from build123d import *

# Parameters (mm, degrees)
BOSS_EXTRUDE1_DEPTH     = 9.525
FILLET1_R               = 25.4
BOSS_EXTRUDE2_DEPTH     = 19.05
FILLET2_R               = 6.35
CUT_EXTRUDE1_DEPTH      = 7.9375
SKETCH9_R               = 14.2875
CUT_EXTRUDE3_DEPTH      = 10.525
CUT_EXTRUDE3_DEPTH_BACK = 10.525


with BuildPart() as part:
    # Sketch1 → Boss-Extrude1 (new body, symmetric)
    with BuildSketch(Plane(origin=(0, 0, 0), x_dir=(0, 0, -1), z_dir=(1, 0, 0))):
        Polygon((0, 0), (0, -112.563749307), (261.582885953, -457.593888215), (450.85, -457.593888215), (450.85, 690.679166755), (208.861297127, 733.352902663), (171.366736958, 520.733599781), (293.482501466, 499.198975136), (217.390599948, 67.706860465), (221.513774593, 49.108421529), align=None)
    extrude(amount=BOSS_EXTRUDE1_DEPTH, both=True)

    # Fillet1
    fillet1_edges = [part.edges().sort_by_distance(p)[0] for p in [
        (0, 499.198975136, -293.482501466),
        (0, 520.733599781, -171.366736958),
        (0, 733.352902663, -208.861297127),
        (0, 690.679166755, -450.85),
        (0, -457.593888215, -450.85),
        (0, -457.593888215, -261.582885953),
        (0, -112.563749307, 0),
    ]]
    fillet(fillet1_edges, radius=FILLET1_R)

    # Sketch5 → Boss-Extrude2 (add)
    with BuildSketch(Plane(origin=(9.525, 0, 0), x_dir=(0, 0, -1), z_dir=(1, 0, 0))):
        Polygon((24.797918581, 5.497566194), (23.079929145, 13.246915751), (147.069522049, 40.734746721), (148.787511485, 32.985397164), align=None)
    extrude(amount=-BOSS_EXTRUDE2_DEPTH)

    # Fillet2
    fillet2_edges = [part.edges().sort_by_distance(p)[0] for p in [
        (0, 32.985397164, -148.787511485),
        (0, 5.497566194, -24.797918581),
    ]]
    fillet(fillet2_edges, radius=FILLET2_R)

    # Sketch6 → Cut-Extrude1 (cut)
    with BuildSketch(Plane(origin=(9.525, 0, 0), x_dir=(0, 0, -1), z_dir=(1, 0, 0))):
        with BuildLine():
            Line((28.6385, -6.365075015), (28.6385, -100.980075015))
            ThreePointArc((28.6385, -100.980075015), (20.574, -109.044575015), (12.5095, -100.980075015))
            Line((12.5095, -100.980075015), (12.5095, -6.365075015))
            ThreePointArc((12.5095, -6.365075015), (20.574, 1.699424985), (28.6385, -6.365075015))
        make_face()
        with BuildLine():
            Line((418.973, -269.390231885), (418.973, 670.409768115))
            ThreePointArc((418.973, 670.409768115), (427.0375, 678.474268115), (435.102, 670.409768115))
            Line((435.102, 670.409768115), (435.102, -269.390231885))
            ThreePointArc((435.102, -269.390231885), (427.0375, -277.454731885), (418.973, -269.390231885))
        make_face()
        with BuildLine():
            Line((354.524032203, 662.256458615), (332.470713639, 537.185873983))
            ThreePointArc((332.470713639, 537.185873983), (323.128345786, 530.644277587), (316.586749391, 539.98664544))
            Line((316.586749391, 539.98664544), (338.640067954, 665.057230073))
            ThreePointArc((338.640067954, 665.057230073), (347.982435807, 671.598826468), (354.524032203, 662.256458615))
        make_face()
        with BuildLine():
            Line((406.559861559, 491.68872453), (197.491872287, 528.553051841))
            ThreePointArc((197.491872287, 528.553051841), (189.629312583, 536.333399232), (194.145410605, 546.430849865))
            Line((194.145410605, 546.430849865), (228.335527156, 740.311741223))
            ThreePointArc((228.335527156, 740.311741223), (231.057354489, 742.217510482), (232.963123748, 739.495683149))
            Line((232.963123748, 739.495683149), (199.190848291, 547.984231028))
            Line((199.190848291, 547.984231028), (409.934019299, 510.824523979))
            ThreePointArc((409.934019299, 510.824523979), (417.814840153, 499.569545384), (406.559861559, 491.68872453))
        make_face()
        with BuildLine():
            Line((250.866088981, 80.873965121), (323.642040242, 493.606894408))
            ThreePointArc((323.642040242, 493.606894408), (317.100443846, 502.949262261), (307.758075993, 496.407665866))
            Line((307.758075993, 496.407665866), (234.982124733, 83.674736578))
            ThreePointArc((234.982124733, 83.674736578), (241.523721128, 74.332368726), (250.866088981, 80.873965121))
        make_face()
        with BuildLine():
            Line((41.2115, -97.692152626), (91.0115, -97.692152626))
            ThreePointArc((91.0115, -97.692152626), (99.076, -105.756652626), (91.0115, -113.821152626))
            Line((91.0115, -113.821152626), (41.2115, -113.821152626))
            ThreePointArc((41.2115, -113.821152626), (33.147, -105.756652626), (41.2115, -97.692152626))
        make_face()
    extrude(amount=-CUT_EXTRUDE1_DEPTH, mode=Mode.SUBTRACT)

    # Sketch9 → Cut-Extrude3 (cut, two sides)
    with BuildSketch(Plane(origin=(0, 0, 0), x_dir=(0, 0, -1), z_dir=(1, 0, 0))) as cut_extrude3_sk:
        with Locations((49.5935, -44.45)):
            Circle(SKETCH9_R)
    extrude(amount=CUT_EXTRUDE3_DEPTH, mode=Mode.SUBTRACT)
    extrude(cut_extrude3_sk.sketch, amount=-CUT_EXTRUDE3_DEPTH_BACK, mode=Mode.SUBTRACT)


solid = part.part
The model under review builds one solid part; all positions refer to its coordinate system, in mm. A direction names the side the tool comes from. Coordinates: 2 decimals unless noted, no trailing zeros. Write each loop counter-clockwise with the first axis right and the second up, starting at its lowest first coordinate (ties: lowest second). Pieces come first, ordered by that corner, then holes. Notation, with made-up numbers: M 35.5,-37.75 L 51.5,-37.75 A19 cw 51.5,-27.75 Z; hole C 46,-31 d10. An arc over 180 degrees is marked long. Put each result on its own line as item: value.
1) Draft analysis for pull direction Z (two halves, no side actions). For faces 4 (the flat face through (-9.525, 144, -272)), 5 (the flat face through (1.588, 290, -279)), 6 (the cylindrical face through (0.13, 685.88, -444.75)), 7 (the flat face through (5.6, 639.9, -215.4)), state which applies: released by +Z, released by -Z, zero draft, split by the parting line, or undercut.
Computed:
face 4: zero draft
face 5: undercut
face 6: released by -Z
face 7: undercut
2) Add section D-D on z = -132. Give the boundary of the cut face in (x, y) (3 decimals).
Computed:
outline: M -9.525,-286.673 L 9.525,-286.673 L 9.525,37.394 L -9.525,37.394 Z
3) Clearance check with flat-ended pins moving along their axes: pin 1 Ø2.5 at (x, z) = (5.5, -69) entering from -Y; pin 2 Ø4 at (x, z) = (-0.5, -325) entering from +Y (3 decimals); pin 3 Ø8 at (x, z) = (-4, -165) entering from +Y. State where each tip first meets the part, or that it passes through.
Computed:
pin 1: stops at y = -205.22
pin 2: stops at y = 713.225
pin 3: stops at y = 37.47
4) For faces 1 (the flat face through (0.133, 510.055, -231.92)), 2 (the flat face through (5.61, 601.65, -327.46)), 3 (the flat face through (0.133, 628.181, -190.315)), list the 3-axis set-ups (+Z, -Z, +X, -X, +Y, -Y) from which the entire face can be reached by the end or side of a thin tool; tool diameter is ignored.
Computed:
face 1: +Z, +X, -X
face 2: +X
face 3: +Z, +X, -X, +Y
5) Wall thickness on probe 1 along Z at (x, y) = (3.5, -44.45); probe 2 along Z at (x, y) = (6.25, 575); probe 3 along Z at (x, y) = (3, 284): over which ranges is each line inside the solid? List them lowest first. Write a range as [from, to].
Computed:
probe 1: z = [-450.85, -435.1], [-418.97, -63.88], [-35.31, -28.64], [-12.51, 0]
probe 2: z = [-450.85, -435.1], [-418.97, -339.14], [-322.76, -203.95], [-199.18, -180.94]
probe 3: z = [-450.85, -435.1], [-418.97, -286.68], [-270.3, -255.53]
